Here's how the part is built. I have some questions about the finished solid (model axes, mm). A direction names the side the tool comes from. Round coordinates to 2 decimals unless told otherwise and drop trailing zeros. Write item = value, one per line. Start each with the question number.
Item 1: Which directions (+Z, -Z, +X, -X, +Y, -Y) give clear straight access to the entire face, cutting with the end or side of a thin tool? Please do faces 1 (the face through (42.52, 2.21, 1.01)), 2 (the face through (-1, -14.8, 1)), 3 (the face through (21, 26, 6)), 4 (the face through (15.1, 26, 6)).
Item 2: For P1, Ø1.2, axis at x = 6, z = 1, coming from the +Y side; P2, Ø10, axis at x = -17, y = -19.5, coming from the +Z side; P3, Ø0.8, axis at y = 26, z = 6, coming from the +X side, each with a flat end and sliding along its axis, tell me the tip position at first contact or that it passes through.
Item 3: If I drill on line 1 along X through (y, z) = (24.5, 4.9); line 2 along Y through (x, z) = (-40.05, 5.3); line 3 along Y through (x, z) = (-40.05, 3.5), over which ranges is the centre line in solid material (lowest first)? Write a range as [from, to].
Item 4: If we section it at A-A (x = 17.95): Give the number of separate pieces and of enclosed holes in the cut face, and give its area (3 significant figures).
Item 5: Thinking about a two-plate mould opening in Y: for faces 5 (the face through (-9.65, -26.99, 0.98)), 6 (the face through (-1, 19.2, 1)), 7 (the face through (42.52, -1.79, 1.01)), which applies, pulls with the +Y half, pulls with the -Y half, needs draft (parallel to the pull), parting line crosses it, or undercut?
```python
from build123d import *

# Parameters (mm, degrees)
PAD_DEPTH           = 4.5
SKETCH001_W         = 5.9
SKETCH001_H         = 6.5
PAD001_DEPTH        = 2.7
SKETCH002_W         = 87
SKETCH002_H         = 2
POCKET_DEPTH        = 2.5
LINEARPATTERN_COUNT = 11
LINEARPATTERN_PITCH = 4
SKETCH003_W         = 4.9
SKETCH003_H         = 7.2
POCKET001_DEPTH     = 2.1
SKETCH004_R         = 1.35
POCKET002_DEPTH     = 212.531374
CHAMFER_SIZE        = 1.99
POCKET003_DEPTH     = 2.7
SKETCH006_W         = 11.5
SKETCH006_H         = 11.5
PAD002_DEPTH        = 1.3


with BuildPart() as part:
    # Sketch → Pad (new body)
    with BuildSketch(Plane.XY):
        with BuildLine():
            Line((43.5, 25), (43.5, -25))
            ThreePointArc((40.5, -28), (42.62132, -27.12132), (43.5, -25))
            Line((-40.5, -28), (40.5, -28))
            ThreePointArc((-43.5, -25), (-42.62132, -27.12132), (-40.5, -28))
            Line((-43.5, -25), (-43.5, 25))
            ThreePointArc((-40.5, 28), (-42.62132, 27.12132), (-43.5, 25))
            Line((-40.5, 28), (40.5, 28))
            ThreePointArc((43.5, 25), (42.62132, 27.12132), (40.5, 28))
        make_face()
    extrude(amount=PAD_DEPTH)

    # Sketch001 (on Face10 of Pad) → Pad001 (join)
    with BuildSketch(Plane.XY.offset(4.5)):
        with BuildLine():
            Line((-43.5, 21.5), (-37, 21.5))
            Line((-37, 21.5), (-37, 28))
            Line((-37, 28), (-40.5, 28))
            ThreePointArc((-40.5, 28), (-42.62132, 27.12132), (-43.5, 25))
            Line((-43.5, 21.5), (-43.5, 25))
        make_face()
        with Locations((18.05, 24.75)):
            Rectangle(SKETCH001_W, SKETCH001_H)
        with BuildLine():
            Line((-43.5, -21.5), (-43.5, -25))
            ThreePointArc((-43.5, -25), (-42.62132, -27.12132), (-40.5, -28))
            Line((-40.5, -28), (-37, -28))
            Line((-37, -21.5), (-37, -28))
            Line((-43.5, -21.5), (-37, -21.5))
        make_face()
        with Locations((18.05, -24.75)):
            Rectangle(SKETCH001_W, SKETCH001_H)
    extrude(amount=PAD001_DEPTH)

    # Sketch002 (on Face4 of Pad001) → Pocket (cut)
    with BuildSketch(Plane(origin=(0, 0, 0), x_dir=(1, 0, 0), z_dir=(0, 0, -1))):
        with Locations((0, 19.8)):
            Rectangle(SKETCH002_W, SKETCH002_H)
    pocket = extrude(amount=-POCKET_DEPTH, mode=Mode.SUBTRACT)

    # LinearPattern: Pocket ×11
    with Locations(*[(0, i * LINEARPATTERN_PITCH, 0) for i in range(1, LINEARPATTERN_COUNT)]):
        add(pocket, mode=Mode.SUBTRACT)

    # Sketch003 (on Face26 of LinearPattern) → Pocket001 (cut)
    with BuildSketch(Plane(origin=(0, 0, 0), x_dir=(1, 0, 0), z_dir=(0, 0, -1))):
        with BuildLine():
            Line((-43.5, 25), (-43.5, 20.8))
            Line((-43.5, 20.8), (-34.1, 20.8))
            Line((-34.1, 20.8), (-34.1, 28))
            Line((-40.5, 28), (-34.1, 28))
            ThreePointArc((-40.5, 28), (-42.62132, 27.12132), (-43.5, 25))
        make_face()
        with Locations((17.95, 24.4)):
            Rectangle(SKETCH003_W, SKETCH003_H)
    pocket001 = extrude(amount=-POCKET001_DEPTH, mode=Mode.SUBTRACT)

    # Mirrored: Pocket001 across Sketch003 H_Axis
    add(pocket001.mirror(Plane(origin=(0, 0, 0), x_dir=(0, 0, -1), z_dir=(0, -1, 0))), mode=Mode.SUBTRACT)

    # Sketch004 (on Face33 of Mirrored) → Pocket002 (cut, through all)
    with BuildSketch(Plane(origin=(0, 0, 2.1), x_dir=(1, 0, 0), z_dir=(0, 0, -1))):
        with Locations((-40.05, 24.5)):
            Circle(SKETCH004_R)
        with Locations((17.95, 24.5)):
            Circle(SKETCH004_R)
    pocket002 = extrude(amount=-POCKET002_DEPTH, mode=Mode.SUBTRACT)

    # Mirrored001: Pocket002 across Sketch004 H_Axis
    add(pocket002.mirror(Plane(origin=(0, 0, 2.1), x_dir=(0, 0, -1), z_dir=(0, -1, 0))), mode=Mode.SUBTRACT)

    # Chamfer
    chamfer_edges = [part.edges().sort_by_distance(p)[0] for p in [
        (-9.3, 28, 0),
        (-43.5, 18.2, 0),
        (-43.5, 14.2, 0),
        (-43.5, 10.2, 0),
        (-43.5, 6.2, 0),
        (-43.5, 2.2, 0),
        (-43.5, -1.8, 0),
        (-43.5, -5.8, 0),
        (-43.5, -9.8, 0),
        (-43.5, -13.8, 0),
        (-43.5, -17.8, 0),
        (-9.3, -28, 0),
        (30.45, -28, 0),
        (42.62132, -27.12132, 0),
        (43.5, -22.9, 0),
        (43.5, -17.8, 0),
        (43.5, -13.8, 0),
        (43.5, -9.8, 0),
        (43.5, -5.8, 0),
        (43.5, -1.8, 0),
        (43.5, 2.2, 0),
        (43.5, 6.2, 0),
        (43.5, 10.2, 0),
        (43.5, 14.2, 0),
        (43.5, 18.2, 0),
        (43.5, 23.1, 0),
        (42.62132, 27.12132, 0),
        (30.45, 28, 0),
    ]]
    chamfer(chamfer_edges, length=CHAMFER_SIZE)

    # Sketch005 (on Face21 of Chamfer) → Pocket003 (cut)
    with BuildSketch(Plane.XY.offset(7.2)):
        with BuildLine():
            Line((-40, 21.5), (-37, 21.5))
            Line((-37, 24.5), (-37, 21.5))
            ThreePointArc((-40, 21.5), (-37.87868, 22.37868), (-37, 24.5))
        make_face()
        with BuildLine():
            Line((15.1, 21.5), (21, 21.5))
            Line((21, 24.458305), (21, 21.5))
            ThreePointArc((15.1, 24.458305), (18.05, 21.508305), (21, 24.458305))
            Line((15.1, 21.5), (15.1, 24.458305))
        make_face()
    pocket003 = extrude(amount=-POCKET003_DEPTH, mode=Mode.SUBTRACT)

    # Mirrored002: Pocket003 across Sketch005 H_Axis
    add(pocket003.mirror(Plane(origin=(0, 0, 7.2), x_dir=(0, 0, 1), z_dir=(0, 1, 0))), mode=Mode.SUBTRACT)

    # Sketch006 (on Face110 of Mirrored002) → Pad002 (join)
    with BuildSketch(Plane.XY.offset(4.5)):
        with Locations((-0.05, 5.65)):
            Rectangle(SKETCH006_W, SKETCH006_H)
    extrude(amount=PAD002_DEPTH)


solid = part.part
```
Reply:
q1.face_1 = -Z, +X, +Y, -Y
q1.face_2 = -Z, +X, -X
q1.face_3 = +Z, +X, +Y, -Y
q1.face_4 = +Z, +Y, -Y
q2.P1 = 27.61
q2.P2 = 4.5
q2.P3 = 21
q3.line_1 = [-43.5, -41.4], [-38.7, -37], [15.1, 16.6], [19.3, 21]
q3.line_2 = [-28, -25.85], [-23.15, -21.5], [21.5, 23.15], [25.85, 28]
q3.line_3 = [-28, -25.85], [-23.15, 23.15], [25.85, 28]
q4.separate_pieces = 3
q4.enclosed_holes = 0
q4.area = 175 mm2
q5.face_5 = pulls with the -Y half
q5.face_6 = undercut
q5.face_7 = needs draft
